from build123d import *

# Parameters (mm, degrees)
ESQUISSE4_R                     = 2
ENL_V_MAT_EXTRU_1_DEPTH         = 10
R_P_TITION_CIRCULAIRE1_COUNT    = 2
ENL_V_START                     = -1
ENL_V_DE_MAT_EXTRU_MINCE1_DEPTH = 1


# Read off the part's stored shape, not the designer's step: Enlèv. de mat.-Extru.-Mince1
with BuildPart() as part:
    # Esquisse3 → Révolution5 (revolve)
    with BuildSketch(Plane.XY, mode=Mode.PRIVATE) as r_volution5_sk:
        with BuildLine():
            Line((14, -7.071067812), (14, -15))
            Line((14, -15), (0, -15))
            Line((0, -15), (0, -25))
            Line((0, -25), (-1, -25))
            Line((-1, -25), (-1, 0))
            Line((-1, 0), (19, 0))
            ThreePointArc((19, 0), (17.623724357, -4.330127019), (14, -7.071067812))
        make_face()
    revolve(r_volution5_sk.sketch.rotate(Axis((-63.101738984, 0, 0), (1, 0, 0)), 270), axis=Axis((-63.101738984, 0, 0), (1, 0, 0)))

    # Esquisse4 → Enlèv. mat.-Extru.1 (cut)
    with BuildSketch(Plane(origin=(0, 0, 0), x_dir=(0, 0, -1), z_dir=(1, 0, 0))):
        with Locations((17.167855519, 10.259860471)):
            Circle(ESQUISSE4_R)
    enl_v_mat_extru_1 = extrude(amount=-ENL_V_MAT_EXTRU_1_DEPTH, mode=Mode.SUBTRACT)

    # Répétition circulaire1: Enlèv. mat.-Extru.1 ×2 about axis
    r_p_tition_circulaire1_axis = Axis((0, 0, 0), (1, 0, 0))
    for i in range(1, R_P_TITION_CIRCULAIRE1_COUNT):
        add(enl_v_mat_extru_1.rotate(r_p_tition_circulaire1_axis, i * 360 / R_P_TITION_CIRCULAIRE1_COUNT), mode=Mode.SUBTRACT)

    # Enlèv. de mat.-Extru.-Mince1 outline → Enlèv. de mat.-Extru.-Mince1 (cut)
    with BuildSketch(Plane(origin=(0, 0, 0), x_dir=(0, 0, -1), z_dir=(1, 0, 0)).offset(ENL_V_START)):
        with BuildLine():
            ThreePointArc((-21.459819345, -12.824825678), (-21.528104694, -7.812775037), (-17.214284766, -5.260076044))
            ThreePointArc((-17.214284766, -5.260076044), (-13.162462305, 12.278012301), (4.051895913, 17.538019829))
            ThreePointArc((4.051895913, 17.538019829), (4.037882143, 17.51270813), (4.02391722, 17.487369448))
            Line((4.02391722, 17.487369448), (12.786542752, 12.66903013))
            Line((12.786542752, 12.66903013), (14.799239297, 14.663229317))
            ThreePointArc((14.799239297, 14.663229317), (18.49817446, 15.079637594), (21.459819345, 12.824825678))
            ThreePointArc((21.459819345, 12.824825678), (-12.824825678, 21.459819345), (-21.459819345, -12.824825678))
        make_face()
        with BuildLine():
            ThreePointArc((-14.799239297, -14.663229317), (-18.49817446, -15.079637594), (-21.459819345, -12.824825678))
            ThreePointArc((-21.459819345, -12.824825678), (12.824825678, -21.459819345), (21.459819345, 12.824825678))
            ThreePointArc((21.459819345, 12.824825678), (21.528104694, 7.812775037), (17.214284766, 5.260076044))
            ThreePointArc((17.214284766, 5.260076044), (13.162462305, -12.278012301), (-4.051895913, -17.538019829))
            ThreePointArc((-4.051895913, -17.538019829), (-4.037882143, -17.51270813), (-4.02391722, -17.487369448))
            Line((-4.02391722, -17.487369448), (-12.786542752, -12.66903013))
            Line((-12.786542752, -12.66903013), (-14.799239297, -14.663229317))
        make_face()
    extrude(amount=ENL_V_DE_MAT_EXTRU_MINCE1_DEPTH, mode=Mode.SUBTRACT)


solid = part.part
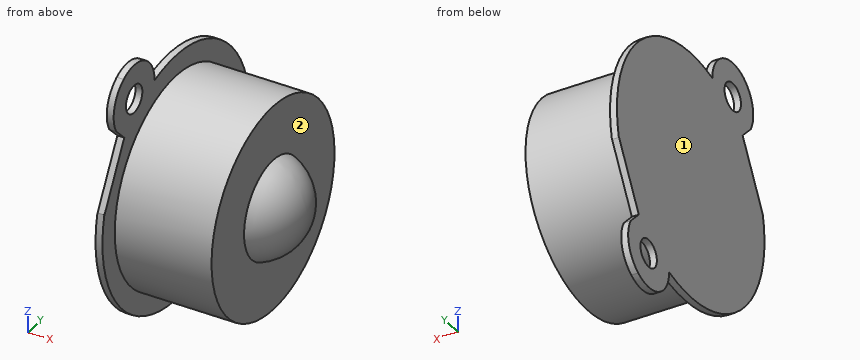
Geometry check sheet. Reference: the model listing, model coordinates, mm. Face numbers are marked on the shaded views. A direction names the side the tool comes from. Coordinates: 2 decimals unless noted, no trailing zeros. Order: outer loops, then holes, each group sorted by start corner. A loop starts at its lowest first (then second) coordinate and runs counter-clockwise, first axis right, second up. Notation, with made-up numbers: (-39.75, 42) - (19.25, 42) arc R17 ccw to (19.25, 73) - close; hole circle Ø5 at (7.25, -33). An arc over 180 degrees is marked (long way). One line per item, written item: value.
(1) Sectioned sample at B-B (z = -1). Enter the section's corners in (x, y).
Data:
outline: (-1, -17.97) - (0, -17.97) - (0, -14.97) - (14, -14.97) - (14, -7) arc R7.43 ccw to (14, 7) - (14, 14.97) - (0, 14.97) - (0, 17.97) - (-1, 17.97) - close
(2) Depth check by flat-ended pin: pin 1 Ø5 at (x, z) = (13.5, -5) entering from +Y; pin 2 Ø12 at (x, y) = (14, -14) entering from -Z; pin 3 Ø10 at (x, y) = (9.5, 2.5) entering from +Z; pin 4 Ø3.5 at (y, z) = (-10.26, 17.17) entering from +X. Enter the tip coordinate at first touch or a pass-through.
Data:
pin 1: stops at y = 14.79
pin 2: stops at z = -12.69
pin 3: stops at z = 15
pin 4: passes through
(3) Thickness scan on probe 1 along X at (y, z) = (2.5, -8); probe 2 along X at (y, z) = (-10, 13.5); probe 3 along Y at (x, z) = (13, -8.5). Record the ranges inside material, lowest first. Write a range as from..to.
Data:
probe 1: x = -1..14
probe 2: x = -1..0
probe 3: y = -12.36..12.36
(4) Sectioned sample at A-A (y = 0). Enter the section's corners in (x, z).
Data:
outline: (-1, -18) - (0, -18) - (0, -15) - (14, -15) - (14, -7.07) arc R7.5 ccw to (14, 7.07) - (14, 15) - (0, 15) - (0, 18) - (-1, 18) - close
(5) Access from +Z, -Z, +X, -X, +Y, -Y to the whole of each face (thin tool, end or side, straight path). Record for the marked faces 1 and 2.
Data:
face 1: +Z, -Z, -X, +Y, -Y
face 2: +X
(6) Sectioned sample at C-C (x = 11.75). Enter the section's corners in (y, z), and give its area (3 significant figures).
Data:
outline: circle Ø30 at (0, 0)
area: 707 mm^2
(7) Sectioned sample at D-D (x = 16). Enter the section's corners in (y, z).
Data:
outline: circle Ø12 at (0, 0)
